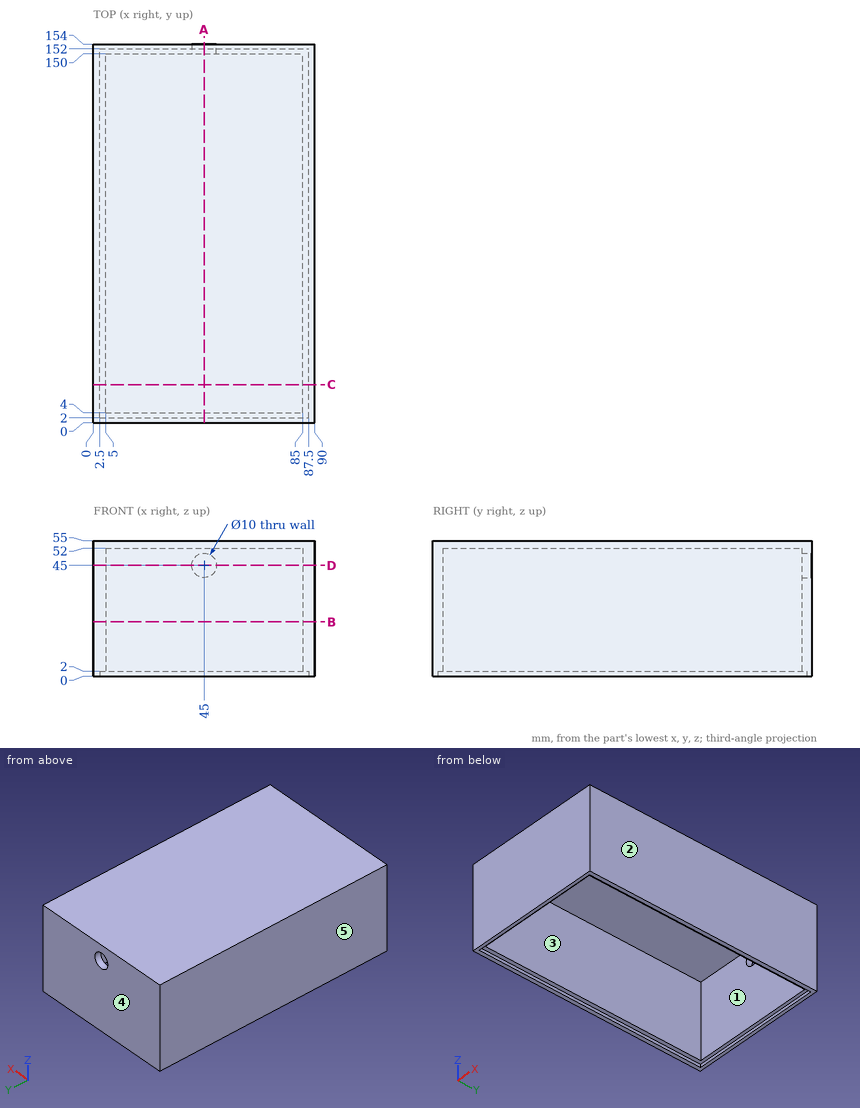
Could you check a few things on this drawing? It's one solid part, dimensions in mm from its lowest x, y, z. A direction names the side the tool comes from. Give positions to 0.01 mm unless a question says otherwise; leave off trailing zeros. Order: outer loops, then holes, each group sorted by start corner. A loop starts at its lowest first (then second) coordinate and runs counter-clockwise, first axis right, second up. Notation, with made-up numbers: (7.25, -32.5) - (28.25, -32.5) arc R17 ccw to (28.25, -2.5) - close; hole circle Ø11 at (3.25, -16). An arc over 180 degrees is marked (long way). One line per question, with ' | ' between items. Start each with the question number.
Item 1: I need wall thicknesses on probe 1 along Y at (x, z) = (69, 21.5); probe 2 along X at (y, z) = (11, 8.5); probe 3 along Z at (x, y) = (45, 151.3). Which ranges of each line are inside material? Lowest first, please. Write a range as [from, to].
Item 2: Thinking about a two-plate mould opening in X: for the marked faces 3, 4 and 5, which applies, pulls with the +X half, pulls with the -X half, needs draft (parallel to the pull), parting line crosses it, or undercut?
Item 3: I want a section at B-B on z = 22. Write out the boundary of the cut face in (x, y), then the cut area to 3 significant figures.
Item 4: For the marked faces 1 and 2, which set-ups out of +Z, -Z, +X, -X, +Y, -Y let a thin tool reach every point of the face, with its end or its side?
Item 5: I want a section at D-D on z = 45. Write out the boundary of the cut face in (x, y), then the cut area to 3 significant figures.
Item 6: I want a section at C-C on y = 15.5. Write out the boundary of the cut face in (x, z), then the cut area to 3 significant figures.
Item 7: I'm going to push a flat-ended pin straight in: pin 1 Ø1 at (x, y) = (35.5, 25.5) entering from -Z. Where does the tip first touch, or does it pass through?
Item 8: I want a section at A-A on x = 45. Write out the boundary of the cut face in (y, z), then the cut area to 3 significant figures.
Verdict:
1) probe 1: [0, 4], [150, 154] | probe 2: [0, 5], [85, 90] | probe 3: [2, 40], [50, 55]
2) face 3: undercut | face 4: needs draft | face 5: pulls with the -X half
3) outline: (0, 0) - (90, 0) - (90, 154) - (0, 154) - close; hole (5, 4) - (85, 4) - (85, 150) - (5, 150) - close | area: 2,180 mm^2
4) face 1: -Z | face 2: +Z, -Z, +X, +Y, -Y
5) outline: (0, 0) - (90, 0) - (90, 154) - (50, 154) - (50, 150) - (85, 150) - (85, 4) - (5, 4) - (5, 150) - (40, 150) - (40, 154) - (0, 154) - close | area: 2,140 mm^2
6) outline: (0, 0) - (2.5, 0) - (2.5, 2) - (5, 2) - (5, 52) - (85, 52) - (85, 2) - (87.5, 2) - (87.5, 0) - (90, 0) - (90, 55) - (0, 55) - close | area: 780 mm^2
7) pin 1: z = 52
8) outline: (0, 0) - (2, 0) - (2, 2) - (4, 2) - (4, 52) - (150, 52) - (150, 50) - (154, 50) - (154, 55) - (0, 55) - close; (150, 2) - (152, 2) - (152, 0) - (154, 0) - (154, 40) - (150, 40) - close | area: 830 mm^2
